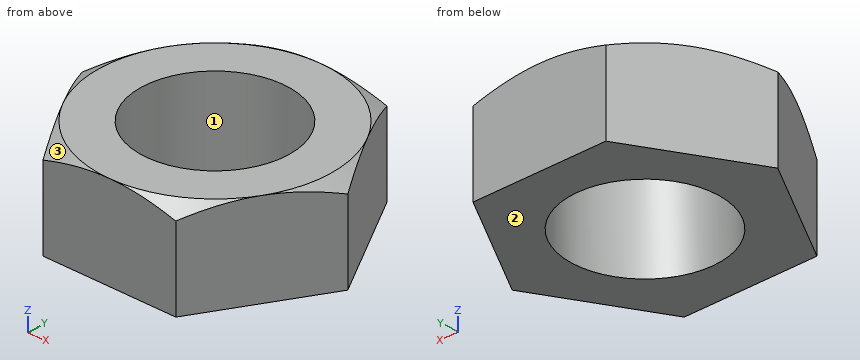
```python
from build123d import *

# Parameters (mm, degrees)
Y_KSEKLIK_EKSTR_ZYON1_DEPTH = 10
IZIM2_R                     = 8
KES_EKSTR_ZYON1_DEPTH       = 10
IZIM3_OUTSIDE_W             = 73.404
IZIM3_OUTSIDE_H             = 69.536
IZIM3_OUTSIDE_R             = 12.5
KES_EKSTR_ZYON2_DEPTH       = 10
KES_EKSTR_ZYON2_DRAFT       = -60


with BuildPart() as part:
    # Çizim1 → Yükseklik-Ekstrüzyon1 (new body)
    with BuildSketch(Plane.XY):
        Polygon((14.43375673, 0), (7.216878365, 12.5), (-7.216878365, 12.5), (-14.43375673, 0), (-7.216878365, -12.5), (7.216878365, -12.5), align=None)
    extrude(amount=Y_KSEKLIK_EKSTR_ZYON1_DEPTH)

    # Çizim2 → Kes-Ekstrüzyon1 (cut)
    with BuildSketch(Plane.XY.offset(10)):
        Circle(IZIM2_R)
    extrude(amount=-KES_EKSTR_ZYON1_DEPTH, mode=Mode.SUBTRACT)


with BuildPart() as kes_ekstr_zyon2_tool:
    # Çizim3 outside → Kes-Ekstrüzyon2 (with draft: the straight prism first)
    with BuildSketch(Plane.XY.offset(10)):
        Rectangle(IZIM3_OUTSIDE_W, IZIM3_OUTSIDE_H)
        Circle(IZIM3_OUTSIDE_R, mode=Mode.SUBTRACT)
    extrude(amount=-KES_EKSTR_ZYON2_DEPTH)
    # Kes-Ekstrüzyon2: the draft: its side faces are tilted about the plane it starts from
    kes_ekstr_zyon2_sides = [kes_ekstr_zyon2_tool.faces().sort_by_distance(p)[0] for p in [
        (0, -34.768, 5),
        (36.702, 0, 5),
        (0, 34.768, 5),
        (-36.702, 0, 5),
        (-12.5, 0, 5),
    ]]
    draft(kes_ekstr_zyon2_sides, Plane.XY.offset(10), KES_EKSTR_ZYON2_DRAFT)


with BuildPart() as part_1:
    add(part.part)

    # Kes-Ekstrüzyon2: cut by kes_ekstr_zyon2_tool
    add(kes_ekstr_zyon2_tool.part, mode=Mode.SUBTRACT)


solid = part_1.part
```
The listing builds one solid part. Answer for the finished solid, in the listing's coordinates (mm). Face numbers are marked on the shaded views. Coordinates: 2 decimals unless noted, no trailing zeros. Loops run counter-clockwise (first coordinate to the right, second up) from the corner with the lowest first, then second, coordinate; pieces in that order, holes last. Notation, with made-up numbers: (42.25, 6) - (48.25, 6) arc R16 cw to (48.25, 20) - close; hole circle Ø6 at (-10, -18.75). An arc over 180 degrees is marked (long way). Write item = value, one per line.
1) Each of these flat-tipped pins is pushed along its axis until it touches: P1, Ø2, axis at y = -7.5, z = 8.5, coming from the +X side; P2, Ø2, axis at y = 10, z = 5, coming from the +X side. Where does it stop, or does it pass through?
Responses:
P1 = 10.68
P2 = 9.24
2) Determine the mould class of the marked faces 1, 2 and 3 for opening direction Y: pulls with the +Y half, pulls with the -Y half, needs draft (parallel to the pull), parting line crosses it, or undercut.
Responses:
face_1 = undercut
face_2 = needs draft
face_3 = pulls with the -Y half
3) Section A-A (z = 5.5) is taken. Determine the outline of the cut face in (x, y).
Responses:
outline = (-14.43, 0) - (-7.22, -12.5) - (7.22, -12.5) - (14.43, 0) - (7.22, 12.5) - (-7.22, 12.5) - close; hole circle Ø16 at (0, 0)
4) Find the intervals of material crossed by line 1 along Y through (x, z) = (0, 6); line 2 along X through (y, z) = (-1.75, 2.5); line 3 along Y through (x, z) = (4.75, 7.25), in increasing order.
Responses:
line_1 = -12.5 to -8, 8 to 12.5
line_2 = -13.42 to -7.81, 7.81 to 13.42
line_3 = -12.5 to -6.44, 6.44 to 12.5
